Can you work these out from the model? Positions are in its coordinate system, mm. A direction names the side the tool comes from. Give positions to 0.01 mm unless a question says otherwise; leave off trailing zeros. Write each loop counter-clockwise with the first axis right and the second up, starting at its lowest first coordinate (ties: lowest second). Pieces come first, ordered by that corner, then holes.
1. Suppose I cut it at A-A (x = -2). Please give me the cut outline in (y, z).
2. On a 3-axis mill with a long thin cutter (end or side, diameter ignored), from which of +Z, -Z, +X, -X, +Y, -Y can I reach the whole of each face in a straight line? I mean faces 1 (the flat face through (0, -4, 1.88)), 2 (the flat face through (0, -3, 3.16)). Say none if no direction works.
3. Thinking about a two-plate mould opening in Z: for faces 3 (the flat face through (0, -4, 2.86)), 4 (the flat face through (-4.47, -5, 1)), 5 (the flat face through (-5, -5, 0.3)), 6 (the cylindrical face through (4.17, -4.22, 1.55)), which applies, pulls with the +Z half, pulls with the -Z half, needs draft (parallel to the pull), parting line crosses it, or undercut?
4. Suppose I cut it at D-D (x = -4). Please give me the cut outline in (y, z), and give its area (3 significant figures).
5. Suppose I cut it at B-B (y = -1.25). Please give me the cut outline in (x, z), and give its area (3 significant figures).
6. Suppose I cut it at C-C (z = 2.4). Please give me the cut outline in (x, y), and give its area (3 significant figures).
7. If I drill on probe 1 along Z at (x, y) = (1, -3.25); probe 2 along Z at (x, y) = (1, -6); probe 3 along Y at (x, z) = (0.5, 1.4), over which ranges is the centre line in solid material (lowest first)?
8. I'm going to push flat-ended pins straight in: pin 1 (1.3 mm diameter, centred on x = 2, z = 2, fed in from -Y); pin 2 (1 mm diameter, centred on x = 5, z = 1, fed in from +Y). Where does each tip first touch, or does it pass through?
```python
from build123d import *

# Parameters (mm, degrees)
PAD_DEPTH     = 6.5
POCKET_DEPTH  = 3.161
SKETCH002_W   = 0.3
SKETCH002_H   = 0.8
PAD001_DEPTH  = 1.58
SKETCH007_W   = 0.6
SKETCH007_H   = 0.7
SKETCH007_W_2 = 0.56
SKETCH007_W_3 = 0.52
PAD002_DEPTH  = 0.2
PAD003_DEPTH  = 2
PAD004_DEPTH  = 5.7
SKETCH008_W   = 1.42
SKETCH008_H   = 0.8
PAD005_DEPTH  = 0.3
FILLET_R      = 0.2


with BuildPart() as part:
    # Sketch → Pad (new body)
    with BuildSketch(Plane.XZ):
        with BuildLine():
            ThreePointArc((-2.89, 3.16), (-4.47, 1.58), (-2.89, 0))
            Line((-2.89, 0), (2.89, 0))
            ThreePointArc((2.89, 0), (4.47, 1.58), (2.89, 3.16))
            Line((2.89, 3.16), (-2.89, 3.16))
        make_face()
        with BuildLine():
            ThreePointArc((-2.89, 2.86), (-4.17, 1.58), (-2.89, 0.3))
            Line((-2.89, 0.3), (2.89, 0.3))
            ThreePointArc((2.89, 0.3), (4.17, 1.58), (2.89, 2.86))
            Line((2.89, 2.86), (-2.89, 2.86))
        make_face(mode=Mode.SUBTRACT)
    extrude(amount=PAD_DEPTH)

    # Sketch001 (on DatumPlane) → Pocket (cut, through all)
    with BuildSketch(Plane(origin=(0, 0, 3.16), x_dir=(-1, 0, 0), z_dir=(0, 0, 1))):
        Polygon((-2.917, 0), (2.917, 0), (2.275486, 0.326), (-2.275486, 0.326), align=None)
    extrude(amount=-POCKET_DEPTH, mode=Mode.SUBTRACT)

    # Sketch002 (on DatumPlane) → Pad001 (join)
    with BuildSketch(Plane(origin=(0, 0, 0), x_dir=(1, 0, 0), z_dir=(0, 0, -1))):
        with Locations((-4.32, 5)):
            Rectangle(SKETCH002_W, SKETCH002_H)
        with Locations((4.32, 5)):
            Rectangle(SKETCH002_W, SKETCH002_H)
        with Locations((-4.32, 0.4)):
            Rectangle(SKETCH002_W, SKETCH002_H)
        with Locations((4.32, 0.4)):
            Rectangle(SKETCH002_W, SKETCH002_H)
    extrude(amount=-PAD001_DEPTH)

    # Sketch007 → Pad002 (join)
    with BuildSketch(Plane(origin=(0, 0, 0), x_dir=(1, 0, 0), z_dir=(0, 0, -1))):
        with Locations((-2.75, 0.23)):
            Rectangle(SKETCH007_W, SKETCH007_H)
        with Locations((-1.52, 0.23)):
            Rectangle(SKETCH007_W_2, SKETCH007_H)
        with Locations((-0.5, 0.23)):
            Rectangle(SKETCH007_W_3, SKETCH007_H)
        with Locations((2.75, 0.23)):
            Rectangle(SKETCH007_W, SKETCH007_H)
        with Locations((1.52, 0.23)):
            Rectangle(SKETCH007_W_2, SKETCH007_H)
        with Locations((0.5, 0.23)):
            Rectangle(SKETCH007_W_3, SKETCH007_H)
    extrude(amount=-PAD002_DEPTH)

    # Sketch005 (on DatumPlane) → Pad003 (join)
    with BuildSketch(Plane(origin=(0, 0, 0), x_dir=(1, 0, 0), z_dir=(0, 1, 0))):
        with BuildLine():
            ThreePointArc((-2.95, -0.3), (-4.23, -1.58), (-2.95, -2.86))
            Line((-2.95, -2.86), (2.95, -2.86))
            ThreePointArc((2.95, -2.86), (4.23, -1.58), (2.95, -0.3))
            Line((2.95, -0.3), (-2.95, -0.3))
        make_face()
    extrude(amount=-PAD003_DEPTH)

    # Sketch006 (on DatumPlane) → Pad004 (join)
    with BuildSketch(Plane(origin=(0, 0, 0), x_dir=(1, 0, 0), z_dir=(0, 1, 0))):
        with BuildLine():
            ThreePointArc((-2.7, -1.28), (-3, -1.58), (-2.7, -1.88))
            Line((-2.7, -1.88), (2.7, -1.88))
            ThreePointArc((2.7, -1.88), (3, -1.58), (2.7, -1.28))
            Line((2.7, -1.28), (-2.7, -1.28))
        make_face()
    extrude(amount=-PAD004_DEPTH)

    # Sketch008 (on DatumPlane) → Pad005 (join)
    with BuildSketch(Plane(origin=(0, 0, 0), x_dir=(1, 0, 0), z_dir=(0, 0, -1))):
        with Locations((-4.88, 5)):
            Rectangle(SKETCH008_W, SKETCH008_H)
        with Locations((-4.88, 0.4)):
            Rectangle(SKETCH008_W, SKETCH008_H)
        with Locations((4.88, 0.4)):
            Rectangle(SKETCH008_W, SKETCH008_H)
        with Locations((4.88, 5)):
            Rectangle(SKETCH008_W, SKETCH008_H)
    extrude(amount=-PAD005_DEPTH)

    # Fillet
    fillet_edges = [part.edges().sort_by_distance(p)[0] for p in [
        (4.47, -0.4, 0.3),
        (4.47, -5, 0.3),
        (4.17, -0.4, 0),
        (4.17, -5, 0),
        (-4.17, -0.4, 0),
        (-4.17, -5, 0),
        (-4.47, -0.4, 0.3),
        (-4.47, -5, 0.3),
        (-5.59, 0, 0.15),
        (-5.59, -5.4, 0.15),
        (-5.59, -0.8, 0.15),
        (5.59, -5.4, 0.15),
        (5.59, -4.6, 0.15),
        (5.59, 0, 0.15),
        (5.59, -0.8, 0.15),
    ]]
    fillet(fillet_edges, radius=FILLET_R)


solid = part.part
```
Checks:
1. outline: (-6.5, 0) - (-0.33, 0) - (-0.33, 0.3) - (0, 0.3) - (0, 2.86) - (-0.33, 2.86) - (-0.33, 3.16) - (-6.5, 3.16) - (-6.5, 2.86) - (-2, 2.86) - (-2, 1.88) - (-5.7, 1.88) - (-5.7, 1.28) - (-2, 1.28) - (-2, 0.3) - (-6.5, 0.3) - close
2. face 1: -Y
2. face 2: +Z, +X, -X, +Y, -Y
3. face 3: undercut
3. face 4: needs draft
3. face 5: pulls with the +Z half
3. face 6: undercut
4. outline: (-6.5, 0.46) - (0, 0.46) - (0, 2.7) - (-6.5, 2.7) - (-6.5, 2.22) - (-2, 2.22) - (-2, 0.94) - (-6.5, 0.94) - close
4. area: 8.88 mm2
5. outline: (-2.89, 0) - (2.89, 0) arc R1.58 ccw to (2.89, 3.16) - (-2.89, 3.16) arc R1.58 ccw to start
5. area: 26.1 mm2
6. outline: (-4.24, -6.5) - (-3.87, -6.5) - (-3.87, -2) - (3.87, -2) - (3.87, -6.5) - (4.24, -6.5) - (4.24, 0) - (-4.24, 0) - close
6. area: 20.3 mm2
7. probe 1: z = 0 to 0.3, 1.28 to 1.88, 2.86 to 3.16
7. probe 2: z = 0 to 0.3, 2.86 to 3.16
7. probe 3: y = -5.7 to 0
8. pin 1: stops at y = -5.7
8. pin 2: passes through
